from build123d import *


with BuildPart() as f2:
    # F2: sweep along a path in F1
    with BuildLine(Plane.XZ) as f2_path:
        Line((0, 266.9991701841), (865.7673536606, 266.9991701841))
        ThreePointArc((865.7673536606, 266.9991701841), (1132.7665238447, 0), (865.7673536606, -266.9991701841))
        Line((865.7673536606, -266.9991701841), (0, -266.9991701841))
        ThreePointArc((0, -266.9991701841), (-266.9991701841, 0), (0, 266.9991701841))
    # F0 (on Right) → F2 (sweep)
    with BuildSketch(Plane.YZ):
        Polygon((10.0134903274, 250.0092067223), (12.7307107569, 269.8237648334), (12.7307107569, 283.9983403683), (-12.7660859497, 283.9749474953), (-12.7400761126, 269.800395824), (-9.9865012549, 249.9908570736), align=None)
    sweep(path=f2_path.line)


solid = f2.part
Part model, mm, in its own coordinate system. A direction names the side the tool comes from. Coordinates: 2 decimals unless noted, no trailing zeros. Order: outer loops, then holes, each group sorted by start corner. A loop starts at its lowest first (then second) coordinate and runs counter-clockwise, first axis right, second up. Notation, with made-up numbers: M 1.25,-28.75 L 42.25,-28.75 A19 ccw 42.25,-4.75 Z; hole C -23.75,-9 d8. An arc over 180 degrees is marked long. Use a Markdown table: item, result.
(1) Cut at B-B on y = 2.5. Write the cut outline in (x, z), then the cut area to 3 significant figures.
A:
| item | result |
|---|---|
| outline | M 0,-283.99 L 865.77,-283.99 A283.99 ccw 865.77,283.99 L 0,283.99 A283.99 ccw Z; hole M 0,-250 L 865.77,-250 A250 ccw 865.77,250 L 0,250 A250 ccw Z |
| area | 116,000 mm^2 |
(2) Probe L1, parallel to Z at x = 724, y = 1; L2, parallel to Z at x = -76, y = -2.75; L3, parallel to X at y = 7, z = -226. List the from-to ranges inside material, lowest first.
A:
| item | result |
|---|---|
| L1 | z = -283.99 to -250, 250 to 283.99 |
| L2 | z = -273.63 to -238.17, 238.17 to 273.63 |
| L3 | x = -171.98 to -106.9, 972.67 to 1037.74 |
(3) Cut at A-A on x = 727.5. Write the cut outline in (y, z), then the cut area to 3 significant figures.
A:
| item | result |
|---|---|
| outline | M -12.77,-283.97 L 12.73,-284 L 12.73,-269.82 L 10.01,-250.01 L -9.99,-249.99 L -12.74,-269.8 Z; M -12.77,283.97 L -12.74,269.8 L -9.99,249.99 L 10.01,250.01 L 12.73,269.82 L 12.73,284 Z |
| area | 1,620 mm^2 |
(4) Pull direction Z, two halves, no side cores. Call faces 3 (the flat face through (436, 12.731, -275)), 4 (the conical face through (-283.918, -0.196, -6.245)), 5 (the conical face through (1116.66, -10.12, 5.52)): released by +Z, released by -Z, zero draft, split by the parting line, or undercut.
A:
| item | result |
|---|---|
| face 3 | zero draft |
| face 4 | split by the parting line |
| face 5 | undercut |
(5) Flat gauge pins, fed straight in: pin 1 (10 mm diameter, centred on x = -129.5, y = -1, fed in from -Z); pin 2 (1.5 mm diameter, centred on y = -4.5, z = 101.5, fed in from +X); pin 3 (4 mm diameter, centred on y = 8.5, z = -192.5, fed in from -X). Where does each tip first touch, or does it go through?
A:
| item | result |
|---|---|
| pin 1 | stops at z = -255.24 |
| pin 2 | stops at x = 1131.28 |
| pin 3 | stops at x = -210.62 |
(6) Tool access for faces 1 (the conical face through (-250.89, -10.12, -5.52)), 2 (the conical face through (1116.955, 10.183, 5.525)): list every direction of +Z, -Z, +X, -X, +Y, -Y with a clear straight run to the whole face (end or side of a thin tool).
A:
| item | result |
|---|---|
| face 1 | -Y |
| face 2 | +Y |
